Input: dimensioned drawing with shaded views. Units: mm. Origin: part minimum x, y, z. Coordinates: 2 decimals unless noted, no trailing zeros. Write each loop counter-clockwise with the first axis right and the second up, starting at its lowest first coordinate (ties: lowest second). Pieces come first, ordered by that corner, then holes. Notation, with made-up numbers: M 84.5,68 L 91.5,68 A26 cw 91.5,106 Z; hole C -31,86 d9. An arc over 180 degrees is marked long. Use one line per item in the form item = value.
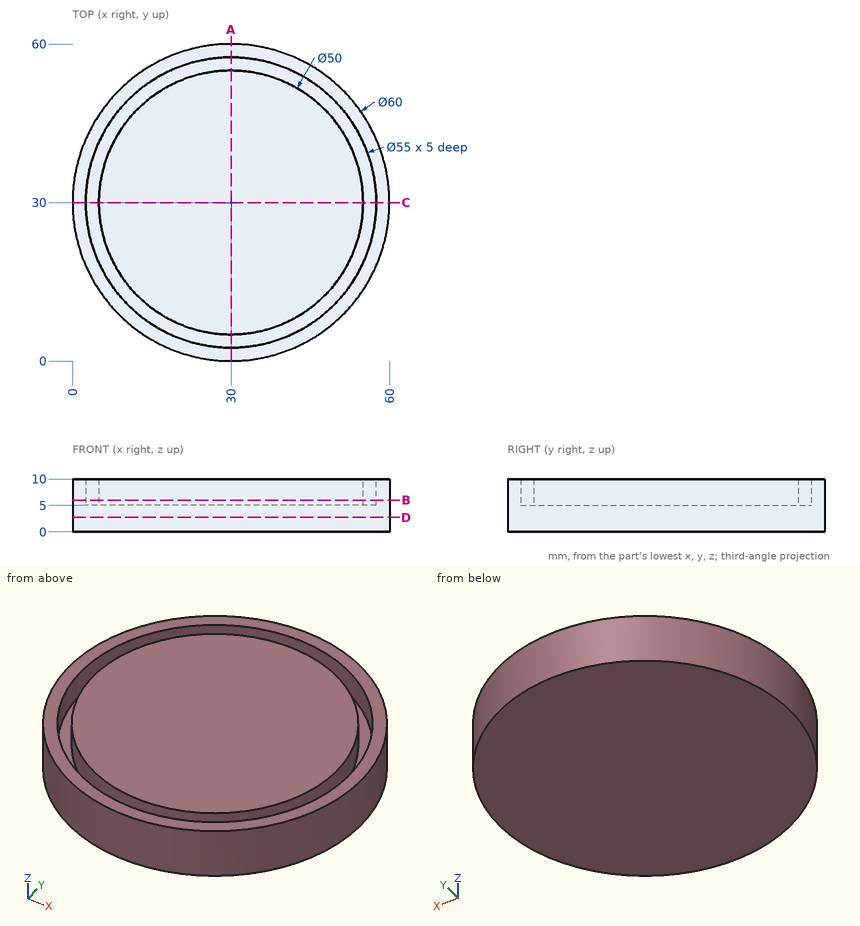
(1) Section query B-B on z = 6. Return the cut outline in (x, y).
Computed:
outline = C 30,30 d60; C 30,30 d50; hole C 30,30 d55
(2) First-contact query: pin 1 Ø1 at (y, z) = (43, 1.5) entering from -X; pin 2 Ø2 at (y, z) = (48.5, 5) entering from -X; pin 3 Ø6 at (x, z) = (47.5, 8) entering from +Y. Flat tips, straight axial feed; report the tip coordinate or a pass-through.
Computed:
pin_1 = 2.73
pin_2 = 5.63
pin_3 = 56.26
(3) Section query A-A on x = 30. Return the cut outline in (y, z).
Computed:
outline = M 0,0 L 60,0 L 60,10 L 57.5,10 L 57.5,5 L 55,5 L 55,10 L 5,10 L 5,5 L 2.5,5 L 2.5,10 L 0,10 Z
(4) Section query D-D on z = 2.75. Return the cut outline in (x, y).
Computed:
outline = C 30,30 d60
(5) Line query: probe 1 along Y at (x, z) = (30, 8.55); probe 2 along Y at (x, z) = (26, 7.75); probe 3 along X at (y, z) = (31, 5.75). Output: solid intervals per line, ascending.
Computed:
probe_1 = 0 to 2.5, 5 to 55, 57.5 to 60
probe_2 = 0.27 to 2.79, 5.32 to 54.68, 57.21 to 59.73
probe_3 = 0.02 to 2.52, 5.02 to 54.98, 57.48 to 59.98
